from build123d import *

# Parameters (mm, degrees)
SKETCH_1_W          = 360
SKETCH_1_H          = 360
EXTRUDE_1_DEPTH     = 20
SKETCH_4_W          = 30
SKETCH_4_H          = 130
EXTRUDE_3_DEPTH     = 25
SKETCH_5_R          = 3
CUT_EXTRUDE_2_DEPTH = 25


with BuildPart() as part:
    # 草图1 → 凸台-拉伸1 (new body)
    with BuildSketch(Plane(origin=(0, 0, 0), x_dir=(1, 0, 0), z_dir=(0, 1, 0))):
        with Locations((180, 180)):
            Rectangle(SKETCH_1_W, SKETCH_1_H)
    extrude(amount=EXTRUDE_1_DEPTH)

    # 草图4 → 凸台-拉伸3 (add)
    with BuildSketch(Plane(origin=(0, 20, 0), x_dir=(1, 0, 0), z_dir=(0, 1, 0))):
        with Locations((345, 295)):
            Rectangle(SKETCH_4_W, SKETCH_4_H)
    extrude(amount=EXTRUDE_3_DEPTH)

    # 草图5 → 切除-拉伸2 (cut)
    with BuildSketch(Plane(origin=(0, 20, 0), x_dir=(1, 0, 0), z_dir=(0, 1, 0))):
        with Locations(Location((15, 110, 0), (0, 0, 270))):
            Circle(SKETCH_5_R)
        with Locations(Location((105, 110, 0), (0, 0, 270))):
            Circle(SKETCH_5_R)
        with Locations(Location((15, 20, 0), (0, 0, 270))):
            Circle(SKETCH_5_R)
        with Locations(Location((105, 20, 0), (0, 0, 270))):
            Circle(SKETCH_5_R)
    extrude(amount=-CUT_EXTRUDE_2_DEPTH, mode=Mode.SUBTRACT)


solid = part.part
Input: part model. Units: mm. Frame: model coordinates. A direction names the side the tool comes from. Coordinates: 2 decimals unless noted, no trailing zeros. Loops run counter-clockwise (first coordinate to the right, second up) from the corner with the lowest first, then second, coordinate; pieces in that order, holes last.
(1) Section A-A on z = -291. Return the cut outline in (x, y).
(2) Material intervals for probe 1 along X at (y, z) = (12, -110); probe 2 along Y at (x, z) = (106, -91.5); probe 3 along X at (y, z) = (31.5, -337), sorted ascending.
(3) Section B-B on y = 25.5. Return the cut outline in (x, z), then the cut area to 3 significant figures.
(4) Set-up query: faces 1 (the face through (177, 0, -183)), 2 (the face through (345, 32, -230)), 3 (the face through (330, 32, -294)). Return all of +Z, -Z, +X, -X, +Y, -Y with unobstructed straight access to the full face (end or side cutting, diameter ignored); none if empty.
(5) Section C-C on x = 216.5. Return the cut outline in (y, z).
(6) First-contact query: pin 1 Ø9.5 at (x, z) = (15, -20) entering from +Y; pin 2 Ø7.5 at (x, y) = (346, 36.5) entering from +Z. Flat tips, straight axial feed; report the tip coordinate or a pass-through.
Data:
1. outline: (0, 0) - (360, 0) - (360, 45) - (330, 45) - (330, 20) - (0, 20) - close
2. probe 1: x = 0 to 12, 18 to 102, 108 to 360
2. probe 2: y = 0 to 20
2. probe 3: x = 330 to 360
3. outline: (330, -360) - (360, -360) - (360, -230) - (330, -230) - close
3. area: 3,900 mm2
4. face 1: +Z, -Z, +X, -X, -Y
4. face 2: +Z, +X, -X, +Y
4. face 3: +Z, -Z, -X, +Y
5. outline: (0, -360) - (20, -360) - (20, 0) - (0, 0) - close
6. pin 1: stops at y = 20
6. pin 2: stops at z = -230
